Design review of the part shown in the three views and the two pictorial views. Dimensions are in mm from the part's minimum x, y and z. A direction names the side the tool comes from. Round coordinates to 2 decimals unless told otherwise and drop trailing zeros. Loops run counter-clockwise (first coordinate to the right, second up) from the corner with the lowest first, then second, coordinate; pieces in that order, holes last. Notation, with made-up numbers: M 61.5,16 L 109.5,16 A16 cw 109.5,36 Z; hole C 86,26 d3. An arc over 180 degrees is marked long. Answer in a Markdown table with one row per item. Add a question column.
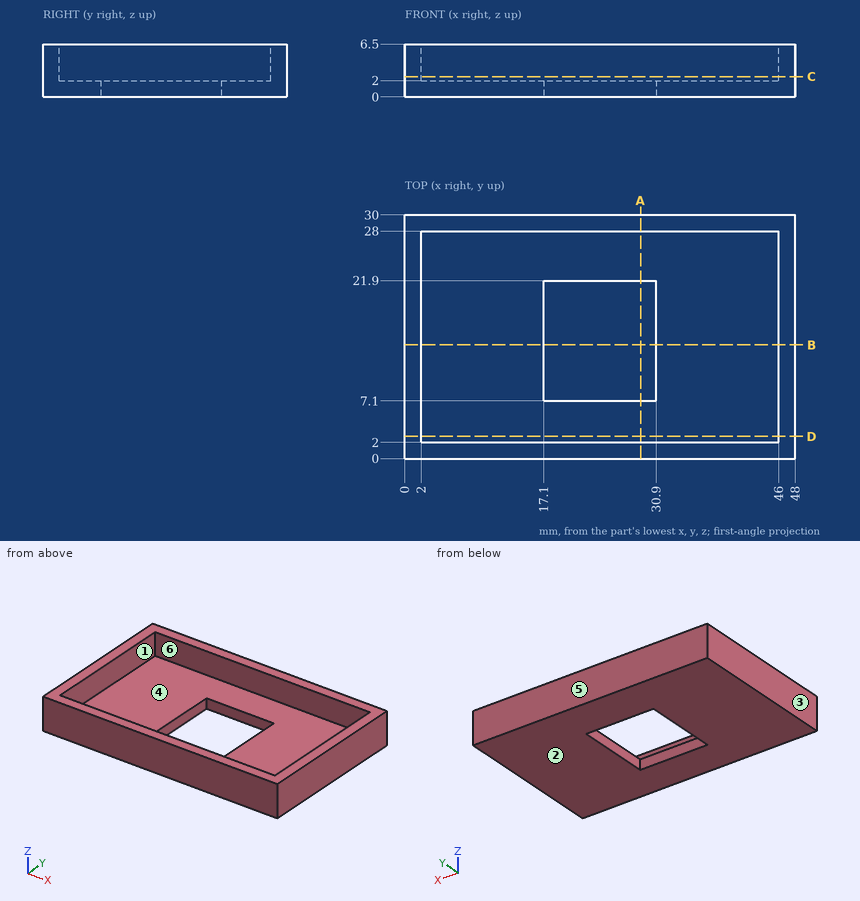
1. Take a section at A-A, the plane x = 29. State the section outline as (y, z) points.
2. Take a section at D-D, the plane y = 2.75. State the section outline as (x, z) points, and give its area (3 significant figures).
3. To check wall thickness, follow probe 1 along Y at (x, z) = (14, 6.25); probe 2 along X at (y, z) = (13.5, 4.25); probe 3 along Z at (x, y) = (26, 6). State the ranges of each line that lie inside material, in increasing order.
4. Machinability: for the marked faces 1 and 2, which of the approach directions +Z, -Z, +X, -X, +Y, -Y give a long, thin tool a straight path to every point of the face, cutting with its end or side? Answer none if there is none.
5. For pin 1 Ø3.5 at (x, z) = (18, 3.5) entering from -Y; pin 2 Ø12 at (x, y) = (15.5, 10.5) entering from +Z, all flat-tipped, find the tip position at first contact; note any pin that passes through.
6. Take a section at B-B, the plane y = 14. State the section outline as (x, z) points, and give its area (3 significant figures).
7. Mouldability with a two-part tool opening along Y and no side actions: class the marked faces 3, 4, 5 and 6 as released by +Y, released by -Y, zero draft, split by the parting line, or undercut.
8. Take a section at C-C, the plane z = 2.5. State the section outline as (x, y) points.
Check sheet entries:
| question | item | result |
|---|---|---|
| 1 | outline | M 0,0 L 7.1,0 L 7.1,2 L 2,2 L 2,6.5 L 0,6.5 Z; M 21.9,0 L 30,0 L 30,6.5 L 28,6.5 L 28,2 L 21.9,2 Z |
| 2 | outline | M 0,0 L 48,0 L 48,6.5 L 46,6.5 L 46,2 L 2,2 L 2,6.5 L 0,6.5 Z |
| 2 | area | 114 mm^2 |
| 3 | probe 1 | y = 0 to 2, 28 to 30 |
| 3 | probe 2 | x = 0 to 2, 46 to 48 |
| 3 | probe 3 | z = 0 to 2 |
| 4 | face 1 | +Z |
| 4 | face 2 | -Z, +X, -X, +Y, -Y |
| 5 | pin 1 | stops at y = 0 |
| 5 | pin 2 | stops at z = 2 |
| 6 | outline | M 0,0 L 17.1,0 L 17.1,2 L 2,2 L 2,6.5 L 0,6.5 Z; M 30.9,0 L 48,0 L 48,6.5 L 46,6.5 L 46,2 L 30.9,2 Z |
| 6 | area | 86.4 mm^2 |
| 7 | face 3 | zero draft |
| 7 | face 4 | undercut |
| 7 | face 5 | released by +Y |
| 7 | face 6 | undercut |
| 8 | outline | M 0,0 L 48,0 L 48,30 L 0,30 Z; hole M 2,2 L 46,2 L 46,28 L 2,28 Z |
